The listing builds one solid part. Answer for the finished solid, in the listing's coordinates (mm). A direction names the side the tool comes from. Round coordinates to 2 decimals unless told otherwise and drop trailing zeros. Order: outer loops, then holes, each group sorted by start corner. A loop starts at its lowest first (then second) coordinate and runs counter-clockwise, first axis right, second up. Notation, with made-up numbers: (16, 67.5) -> (66, 67.5) arc R8 ccw to (66, 72.5) -> close; hole circle Ø10 at (32.25, -39). An arc over 180 degrees is marked (long way). Answer in a Markdown table with one row per item. Add a question column.
```python
from build123d import *

# Parameters (mm, degrees)
SKETCH_R      = 4
PAD_DEPTH     = 4
SKETCH001_R   = 6.5
SKETCH001_R_2 = 4
PAD001_DEPTH  = 4.8
CHAMFER_SIZE  = 0.5
FILLET_R      = 3


with BuildPart() as part:
    # Sketch → Pad (new body)
    with BuildSketch(Plane.XY):
        Polygon((0, 16.5), (-14.289419, 8.25), (-14.289419, -8.25), (0, -16.5), (14.289419, -8.25), (14.289419, 8.25), align=None)
        Circle(SKETCH_R, mode=Mode.SUBTRACT)
    extrude(amount=PAD_DEPTH)

    # Sketch001 (on Face9 of Pad) → Pad001 (join)
    with BuildSketch(Plane.XY.offset(4)):
        Circle(SKETCH001_R)
        Circle(SKETCH001_R_2, mode=Mode.SUBTRACT)
    extrude(amount=PAD001_DEPTH)

    # Chamfer
    chamfer_edges = [part.edges().sort_by_distance(p)[0] for p in [
        (-4, 0, 8.8),
    ]]
    chamfer(chamfer_edges, length=CHAMFER_SIZE)

    # Fillet
    fillet_edges = [part.edges().sort_by_distance(p)[0] for p in [
        (0, -16.5, 2),
        (14.289419, -8.25, 2),
        (14.289419, 8.25, 2),
        (-14.289419, -8.25, 2),
        (-14.289419, 8.25, 2),
        (0, 16.5, 2),
    ]]
    fillet(fillet_edges, radius=FILLET_R)


solid = part.part
```
Item 1: Find the intervals of material crossed by probe 1 along Y at (x, z) = (0, 5.25); probe 2 along Y at (x, z) = (0, 3); probe 3 along Z at (x, y) = (10, 1.5), in increasing order. Write a range as [from, to].
Item 2: For a pull along X with two mould halves and no side action, classify faces 3 (the face through (7.1, -12.4, 2)), 4 (the face through (-0.867, -3.905, 4.092)), 5 (the face through (-4.42, 1.54, 8.8)) as released by +X, released by -X, zero draft, split by the parting line, or undercut.
Item 3: The part is cut by section D-D, the plane z = 7.5. Give the vertices of the cut face in (x, y), and give its area (3 significant figures).
Item 4: A tool of negligible diameter and unlimited length cuts with its end or side. For faces 1 (the face through (-5.158, -3.955, 6.366)), 2 (the face through (-7.22, -12.33, 1.97)), from which of +Z, -Z, +X, -X, +Y, -Y can it reach the whole face along a straight path? Write none if from no direction.
Item 5: The part is cut by section B-B, the plane z = 2.5. Give the vertices of the cut face in (x, y).
Item 6: The part is cut by section A-A, the plane y = 0. Give the vertices of the cut face in (x, z).
Item 7: Flat-ended cylindrical pins translate along their axes: P1, Ø2, axis at x = 2, z = 2, coming from the +Y side; P2, Ø1.5, axis at x = 2.5, z = 3, coming from the +Y side; P3, Ø4, axis at x = 8, y = -2.5, coming from the -Z side; P4, Ø4, axis at y = -9.5, z = 5.5, coming from the +X side. Find the tip coordinate at first contact, or state that the pin passes through.
Item 8: The part is cut by section C-C, the plane x = 0. Give the vertices of the cut face in (y, z).
Resolved:
| question | item | result |
|---|---|---|
| 1 | probe 1 | [-6.5, -4], [4, 6.5] |
| 1 | probe 2 | [-16.04, -4], [4, 16.04] |
| 1 | probe 3 | [0, 4] |
| 2 | face 3 | released by +X |
| 2 | face 4 | undercut |
| 2 | face 5 | zero draft |
| 3 | outline | circle Ø13 at (0, 0); hole circle Ø8 at (0, 0) |
| 3 | area | 82.5 mm2 |
| 4 | face 1 | +Z |
| 4 | face 2 | +Z, -Z, -X, -Y |
| 5 | outline | (-14.29, -6.52) arc R3 ccw to (-12.79, -9.12) -> (-1.5, -15.63) arc R3 ccw to (1.5, -15.63) -> (12.79, -9.12) arc R3 ccw to (14.29, -6.52) -> (14.29, 6.52) arc R3 ccw to (12.79, 9.12) -> (1.5, 15.63) arc R3 ccw to (-1.5, 15.63) -> (-12.79, 9.12) arc R3 ccw to (-14.29, 6.52) -> close; hole circle Ø8 at (0, 0) |
| 6 | outline | (-14.29, 0) -> (-4, 0) -> (-4, 8.3) -> (-4.5, 8.8) -> (-6.5, 8.8) -> (-6.5, 4) -> (-14.29, 4) -> close; (4, 0) -> (14.29, 0) -> (14.29, 4) -> (6.5, 4) -> (6.5, 8.8) -> (4.5, 8.8) -> (4, 8.3) -> close |
| 7 | P1 | y = 15.86 |
| 7 | P2 | y = 15.49 |
| 7 | P3 | z = 0 |
| 7 | P4 | x = 13.79 |
| 8 | outline | (-16.04, 0) -> (-4, 0) -> (-4, 8.3) -> (-4.5, 8.8) -> (-6.5, 8.8) -> (-6.5, 4) -> (-16.04, 4) -> close; (4, 0) -> (16.04, 0) -> (16.04, 4) -> (6.5, 4) -> (6.5, 8.8) -> (4.5, 8.8) -> (4, 8.3) -> close |
